Input: part model. Units: mm. Frame: model coordinates. A direction names the side the tool comes from. Coordinates: 2 decimals unless noted, no trailing zeros. Loops run counter-clockwise (first coordinate to the right, second up) from the corner with the lowest first, then second, coordinate; pieces in that order, holes last. Notation, with made-up numbers: (77, 11.5) -> (94, 11.5) arc R22 ccw to (94, 24.5) -> close; hole circle Ø6 at (58.5, -13.75). An arc over 180 degrees is marked (long way). Put each result on its own line as item: value. Start each with the question number.
1) Set-up query: faces 1 (the flat face through (-42.84, 45.85, 20.94)), 2 (the flat face through (0, 49, -31)), 3 (the flat face through (68.96, 23.74, 29.08)). Return all of +Z, -Z, +X, -X, +Y, -Y with unobstructed straight access to the full face (end or side cutting, diameter ignored); none if empty.
2) Cut plane B-B (y = 20.5). Return the cut outline in (x, z), plus the area to 3 significant figures.
3) Cut plane A-A (z = -7). Return the cut outline in (x, y) (3 decimals), plus the area to 3 significant figures.
4) Material intervals for L1, parallel to X at y = 5.5, z = 16; L2, parallel to X at y = 14, z = -26.5; L3, parallel to X at y = -18, z = 6, sorted ascending.
5) Cut plane C-C (x = 220). Return the cut outline in (y, z), plus the area to 3 significant figures.
6) Contact query for flat-ended pins moving along their axis: P1, Ø1, axis at x = 25.5, z = -9.5, coming from the -Y side; P2, Ø1.5, axis at x = 89.5, z = 18, coming from the +Y side; P3, Ø2, axis at y = 75, z = -27.5, coming from the -X side; P4, Ø12, axis at y = -1.5, z = 4, coming from the -X side. Output: stop coordinate, or through.
7) Pull-direction query (X, two-part tool) for faces 4 (the flat face through (121, 41, 26)), 5 (the flat face through (120, 35, 1)), 6 (the flat face through (113.532, 37.487, -46.576)); classes: pulls with the +X half, pulls with the -X half, needs draft (parallel to the pull), parting line crosses it, or undercut.
8) Cut plane D-D (x = 4). Return the cut outline in (y, z).
from build123d import *

# Parameters (mm, degrees)
BOSS_EXTRUDE1_DEPTH     = 93
BOSS_EXTRUDE2_DEPTH     = 61
BOSS_EXTRUDE3_START     = -25
BOSS_EXTRUDE3_DEPTH     = 62
BOSS_EXTRUDE4_DEPTH     = 2.5
CUT_EXTRUDE2_DEPTH      = 94
CUT_EXTRUDE2_DEPTH_BACK = 26


with BuildPart() as part:
    # Sketch2 → Boss-Extrude1 (new body)
    with BuildSketch(Plane(origin=(0, 0, 0), x_dir=(1, 0, 0), z_dir=(0, 1, 0))):
        Polygon((0, -61), (0, 61), (-93, 0), align=None)
        Polygon((-10, 42.481666483), (-74.767130868, 0), (-10, -42.481666483), align=None, mode=Mode.SUBTRACT)
    extrude(amount=BOSS_EXTRUDE1_DEPTH)

    # Sketch3 → Boss-Extrude2 (add, symmetric)
    with BuildSketch(Plane.XY):
        Polygon((0, 0), (50, 0), (91.711375741, 35), (148.654022129, 35), (199, -25), (244, -25), (244, -19), (201.797845949, -19), (151.451868078, 41), (89.527554335, 41), (47.816178594, 6), (0, 6), align=None)
    extrude(amount=BOSS_EXTRUDE2_DEPTH, both=True)

    # Sketch4 → Boss-Extrude3 (add)
    with BuildSketch(Plane(origin=(0, 0, 0), x_dir=(1, 0, 0), z_dir=(0, 1, 0)).offset(BOSS_EXTRUDE3_START)):
        Polygon((244, -30), (244, 30), (289, 0), align=None)
        Polygon((254, 11.314829082), (270.972243623, 0), (254, -11.314829082), align=None, mode=Mode.SUBTRACT)
    extrude(amount=BOSS_EXTRUDE3_DEPTH)

    # Sketch7 → Boss-Extrude4 (add, symmetric)
    with BuildSketch(Plane.XY):
        Polygon((0, 93), (180.92149546, 93), (227.911074806, 37), (244, 37), (244, -19), (201.797845949, -19), (151.451868078, 41), (89.527554335, 41), (47.816178594, 6), (0, 6), align=None)
    extrude(amount=BOSS_EXTRUDE4_DEPTH, both=True)

    # Sketch8 → Cut-Extrude2 (cut, two sides)
    with BuildSketch(Plane(origin=(0, 0, 0), x_dir=(1, 0, 0), z_dir=(0, 1, 0))) as cut_extrude2_sk:
        Polygon((0, 61), (244, 61), (244, 30), align=None)
        Polygon((0, -61), (244, -30), (244, -61), align=None)
    extrude(amount=CUT_EXTRUDE2_DEPTH, mode=Mode.SUBTRACT)
    extrude(cut_extrude2_sk.sketch, amount=-CUT_EXTRUDE2_DEPTH_BACK, mode=Mode.SUBTRACT)


solid = part.part
Results found:
1. face 1: +Y, -Y
1. face 2: -Z, +Y
1. face 3: +Z, +Y
2. outline: (-93, 0) -> (0, -61) -> (0, -2.5) -> (65.1, -2.5) -> (65.1, -52.73) -> (74.43, -51.54) -> (74.43, 51.54) -> (65.1, 52.73) -> (65.1, 2.5) -> (0, 2.5) -> (0, 61) -> close; (160.82, -40.57) -> (168.65, -39.57) -> (168.65, -2.5) -> (244, -2.5) -> (244, -30) -> (289, 0) -> (244, 30) -> (244, 2.5) -> (168.65, 2.5) -> (168.65, 39.57) -> (160.82, 40.57) -> close; hole (-74.77, 0) -> (-10, -42.48) -> (-10, 42.48) -> close; hole (254, -11.31) -> (270.97, 0) -> (254, 11.31) -> close
2. area: 6,380 mm2
3. outline: (-82.328, 0) -> (-64.095, 0) -> (-64.095, 93) -> (-82.328, 93) -> close; (-10, 0) -> (50, 0) -> (91.711, 35) -> (148.654, 35) -> (199, -25) -> (254, -25) -> (254, 37) -> (244, 37) -> (244, -19) -> (201.798, -19) -> (151.452, 41) -> (89.528, 41) -> (47.816, 6) -> (0, 6) -> (0, 93) -> (-10, 93) -> close; (260.472, -25) -> (278.5, -25) -> (278.5, 37) -> (260.472, 37) -> close
3. area: 6,070 mm2
4. L1: x = -68.61 to -50.37, -10 to 56.55, 173.41 to 181.24, 244 to 265
4. L2: x = -52.6 to -34.37, -10 to 0, 57.35 to 66.68, 166.28 to 174.11, 244 to 249.25
4. L3: x = 193.13 to 200.96, 244 to 254, 261.97 to 280
5. outline: (-25, -33.05) -> (-19, -33.05) -> (-19, -2.5) -> (46.43, -2.5) -> (46.43, 2.5) -> (-19, 2.5) -> (-19, 33.05) -> (-25, 33.05) -> close
5. area: 724 mm2
6. P1: stops at y = 0
6. P2: stops at y = 41
6. P3: stops at x = -52.6
6. P4: stops at x = -93
7. face 4: needs draft
7. face 5: undercut
7. face 6: pulls with the +X half
8. outline: (0, -60.49) -> (6, -60.49) -> (6, -2.5) -> (93, -2.5) -> (93, 2.5) -> (6, 2.5) -> (6, 60.49) -> (0, 60.49) -> close
